from build123d import *

# Parameters (mm, degrees)
F0_R      = 3.175
F0_R_2    = 2.3677964523
F1_DEPTH  = 8.89
F2_W      = 12.7
F2_H      = 6.858
F3_DEPTH  = 8.89
F4_W      = 0.762
F4_H      = 2.032
F5_DEPTH  = 3.937
F7_R      = 3.175
F8_DEPTH  = 1.1684
F11_R     = 1.2243851264
F12_DEPTH = 19.558
F12_TAPER = -2


with BuildPart() as f1:
    # F0 (on Top) → F1 (new body)
    with BuildSketch(Plane.XY):
        Circle(F0_R)
        Circle(F0_R_2, mode=Mode.SUBTRACT)
    extrude(amount=F1_DEPTH)

    # F2 (on face) → F3 (join)
    with BuildSketch(Plane(origin=(0, 0, 0), x_dir=(1, 0, 0), z_dir=(0, 0, -1))):
        Rectangle(F2_W, F2_H)
    extrude(amount=F3_DEPTH)

    # F4 (on face) → F5 (join)
    with BuildSketch(Plane(origin=(0, 0, -8.89), x_dir=(1, 0, 0), z_dir=(0, 0, -1))):
        with Locations((-4.699, 0)):
            Rectangle(F4_W, F4_H)
        Rectangle(F4_W, F4_H)
        with Locations((4.699, 0)):
            Rectangle(F4_W, F4_H)
    extrude(amount=F5_DEPTH)

    # F7 (on offset) → F8 (join)
    with BuildSketch(Plane.XY.offset(3.175)):
        Polygon((-5.297310009, -1.4766115498), (-1.3698718908, -5.3259108144), (3.9274381181, -3.8492992646), (5.297310009, 1.4766115498), (1.3698718908, 5.3259108144), (-3.9274381181, 3.8492992646), align=None)
        Circle(F7_R, mode=Mode.SUBTRACT)
    extrude(amount=F8_DEPTH)

    # F11 (on line) → F12 (join)
    with BuildSketch(Plane(origin=(0, 0, 0), x_dir=(0.9961946981, 0, -0.0871557427), z_dir=(-0.0871557427, 0, -0.9961946981))):
        Circle(F11_R)
    extrude(amount=-F12_DEPTH, taper=F12_TAPER)


solid = f1.part
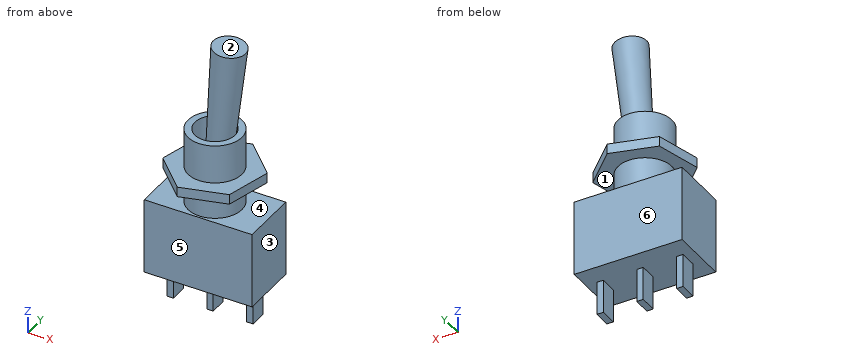
Can you work these out from the model? Positions are in its coordinate system, mm. Face numbers are marked on the shaded views. A direction names the side the tool comes from. Give positions to 0.01 mm unless a question says otherwise; leave off trailing zeros. Loops run counter-clockwise (first coordinate to the right, second up) from the corner with the lowest first, then second, coordinate; pieces in that order, holes last. Notation, with made-up numbers: (79.5, -3.75) -> (131.5, -3.75) arc R17 ccw to (131.5, 7.25) -> close; hole circle Ø2 at (20.5, 60.25). An arc over 180 degrees is marked (long way). Return JSON: item names as keys, results as strings.
Q1. For pin 1 Ø5 at (x, z) = (1, -1) entering from -Y; pin 2 Ø2 at (x, y) = (-1, 1) entering from -Z; pin 3 Ø4 at (x, y) = (4, 4) entering from -Z; pin 4 Ø0.8 at (x, z) = (0, -11) entering from -Y, each with a flat end and sliding along its axis, tell me the tip position at first contact or that it passes through.
Checks:
{"pin 1": "stops at y = -3.43", "pin 2": "stops at z = -12.83", "pin 3": "stops at z = -8.89", "pin 4": "stops at y = -1.02"}
Q2. I want a section at A-A, the plane z = 0.5. Count the separate pieces of the cut face and the enclosed holes in it, then the cut area to 3 significant figures.
Checks:
{"separate pieces": "2", "enclosed holes": "1", "area": "18.9 mm2"}
Q3. We'd pull the mould along Z, two halves only. Please class the marked faces 1, 2 and 3: released by +Z, released by -Z, zero draft, split by the parting line, or undercut.
Checks:
{"face 1": "undercut", "face 2": "released by +Z", "face 3": "zero draft"}
Q4. I need wall thicknesses on probe 1 along Z at (x, y) = (-3.5, 2.75) (3 decimals); probe 2 along Y at (x, z) = (0, 5.75) (3 decimals); probe 3 along Z at (x, y) = (-4.5, 0) (3 decimals). Which ranges of each line are inside material? Lowest first, please.
Checks:
{"probe 1": "z = -8.89 to 0, 3.175 to 4.343", "probe 2": "y = -3.175 to -2.368, -1.333 to 1.333, 2.368 to 3.175", "probe 3": "z = -12.827 to 0, 3.175 to 4.343"}
Q5. On a 3-axis mill with a long thin cutter (end or side, diameter ignored), from which of +Z, -Z, +X, -X, +Y, -Y can I reach the whole of each face in a straight line? I mean the marked faces 4, 5 and 6. Say none if no direction works.
Checks:
{"face 4": "none", "face 5": "-Z, +X, -X, -Y", "face 6": "-Z, +X, -X, +Y"}
Q6. I want a section at B-B, the plane z = -5. List the corners of the cut face in (x, y) for me.
Checks:
{"outline": "(-6.35, -3.43) -> (6.35, -3.43) -> (6.35, 3.43) -> (-6.35, 3.43) -> close"}
